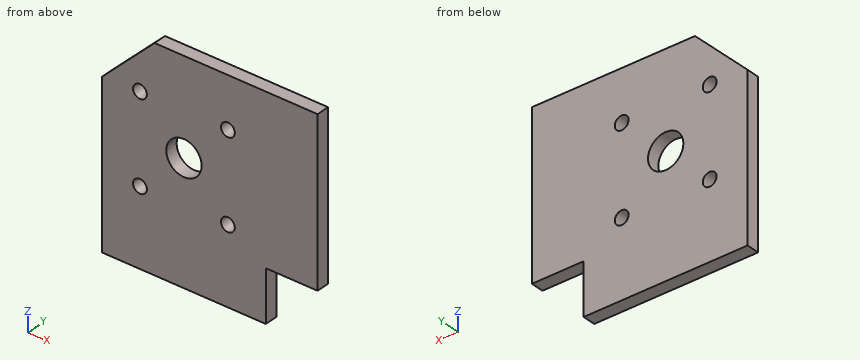
Solid Edge part; units mm, degrees
sketch "Sketch1" plane through (0, 0, 0) normal (0, -1, 0) x (1, 0, 0)
  line L0 (-75.229, -198.7494) -> (174.771, -198.7494)
  line L1 (174.771, -198.7494) -> (174.771, 51.2506)
  line L2 (174.771, 51.2506) -> (-75.229, 51.2506)
  line L3 (-75.229, 51.2506) -> (-75.229, -198.7494)
  dimension "D1" = 75.229
  dimension "D2" = 174.771
extrude "Protrusion1" add sketch "Sketch1" against normal blind 15
sketch "Sketch2" plane through (-15.229, 15, 1.2506) normal (0, 1, 0) x (-1, 0, 0)
  circle A0 centre (16, -111) radius 8
  circle A1 centre (16, -9) radius 8
  circle A2 centre (-86, -111) radius 8
  circle A3 centre (-35, -60) radius 20.5
  circle A4 centre (-86, -9) radius 8
extrude "Cutout1" cut sketch "Sketch2" against normal through all
sketch "Sketch3" plane through (49.771, 0, -73.7494) normal (0, -1, 0) x (-1, 0, 0)
  line L0 (64.0056, -125) -> (125, -64.0056)
  line L1 (125, -64.0056) -> (125, -125)
  line L2 (125, -125) -> (64.0056, -125)
  line L3 (-125, 65) -> (-65, 65)
  line L4 (-65, 65) -> (-65, 125)
  line L5 (-65, 125) -> (-125, 125)
  line L6 (-125, 125) -> (-125, 65)
  dimension "D1" = 125
  dimension "D2" = 125
extrude "Cutout2" cut sketch "Sketch3" against normal through all
properties material "Aluminum, 6061-T6"
Can you work these out from the model? Positions are in its coordinate system, mm. Round coordinates to 2 decimals unless told otherwise and drop trailing zeros. Loops run counter-clockwise (first coordinate to the right, second up) from the corner with the lowest first, then second, coordinate; pieces in that order, holes last. Notation, with made-up numbers: (2, 52) - (45, 52) arc R26 cw to (45, 91) - close; hole circle Ø4 at (33, 37.25). An arc over 180 degrees is marked (long way). Answer in a Markdown table with one row per item. Add a question column.
Q1. I want a section at D-D on y = 5.75. List the corners of the cut face in (x, z) for me.
Q2. I want a section at C-C on x = 73. List the corners of the cut face in (y, z) for me.
Q3. I want a section at B-B on z = -66. List the corners of the cut face in (x, y) for me.
Q4. I want a section at A-A on x = 5. List the corners of the cut face in (y, z) for me, and give its area (3 significant figures).
Q5. I need wall thicknesses on L1, parallel to X at y = 12.75, z = -108; L2, parallel to X at y = 3.5, z = -9.5; L3, parallel to Z at x = 75, y = 7.5. Which ranges of each line are inside material? Lowest first, please.
Q6. For pin 1 Ø7.5 at (y, z) = (4, -181) entering from +X; pin 2 Ø7.5 at (x, y) = (147.5, 4) entering from -Z; pin 3 Ø1.5 at (x, y) = (-38, 12) entering from +Z, each with a flat end and sliding along its axis, tell me the tip position at first contact or that it passes through.
A:
| question | item | result |
|---|---|---|
| 1 | outline | (-75.23, -198.75) - (114.77, -198.75) - (114.77, -138.75) - (174.77, -138.75) - (174.77, 51.25) - (-14.23, 51.25) - (-75.23, -9.74) - close; hole circle Ø16 at (-31.23, -109.75); hole circle Ø16 at (-31.23, -7.75); hole circle Ø41 at (19.77, -58.75); hole circle Ø16 at (70.77, -109.75); hole circle Ø16 at (70.77, -7.75) |
| 2 | outline | (0, -198.75) - (15, -198.75) - (15, -117.43) - (0, -117.43) - close; (0, -102.07) - (15, -102.07) - (15, -15.43) - (0, -15.43) - close; (0, -0.07) - (15, -0.07) - (15, 51.25) - (0, 51.25) - close |
| 3 | outline | (-75.23, 0) - (0.6, 0) - (0.6, 15) - (-75.23, 15) - close; (38.95, 0) - (174.77, 0) - (174.77, 15) - (38.95, 15) - close |
| 4 | outline | (0, -198.75) - (15, -198.75) - (15, -72.96) - (0, -72.96) - close; (0, -44.53) - (15, -44.53) - (15, 51.25) - (0, 51.25) - close |
| 4 | area | 3,320 mm^2 |
| 5 | L1 | -75.23 to -39.04, -23.42 to 62.96, 78.58 to 174.77 |
| 5 | L2 | -74.99 to -39.04, -23.42 to 62.96, 78.58 to 174.77 |
| 5 | L3 | -198.75 to -116.54, -102.96 to -14.54, -0.96 to 51.25 |
| 6 | pin 1 | x = 114.77 |
| 6 | pin 2 | z = -138.75 |
| 6 | pin 3 | z = 28.24 |
